Can you work these out from the model? Positions are in its coordinate system, mm. A direction names the side the tool comes from. Round coordinates to 2 decimals unless told otherwise and drop trailing zeros. Write each loop counter-clockwise with the first axis right and the second up, starting at its lowest first coordinate (ties: lowest second). Pieces come first, ordered by that corner, then holes. Notation, with made-up numbers: M 54,84.5 L 107,84.5 A28 ccw 107,123.5 Z; hole C 29,-15 d5. An arc over 180 degrees is marked long. Answer in a Markdown table with one row per item. Add a question column.
(1) For faces 4 (the face through (10, 0.675, 5)), 5 (the face through (0, -17, 12)), 6 (the face through (-9.4, 1.15, 10)), which set-ups out of +Z, -Z, +X, -X, +Y, -Y let a thin tool reach every point of the face, with its end or its side?
(2) If I drill on probe 1 along Z at (x, y) = (1.75, -4.5); probe 2 along Y at (x, z) = (6.5, 9.5); probe 3 along Y at (x, z) = (4.25, 12.75), over which ranges is the centre line in solid material (lowest first)?
(3) Suppose I cut it at A-A, the plane y = -1.75. Write out the boundary of the cut face in (x, z), then the cut area to 3 significant figures.
(4) I'm going to push flat-ended pins straight in: pin 1 (3.5 mm diameter, centred on x = 10.5, z = 2.5, fed in from -Y); pin 2 (1 mm diameter, centred on x = -6.5, z = 8, fed in from -Y); pin 3 (1.4 mm diameter, centred on x = -11, z = 2.5, fed in from -Y). Where does each tip first touch, or does it pass through?
(5) Suppose I cut it at C-C, the plane z = 1. Write out the boundary of the cut face in (x, y) (3 decimals).
(6) If we mould it in two halves opening along Z, with no side actions, what happens to faces 1 (the face through (0, 2.8, 2)), 2 (the face through (0, -9, 7)), 3 (the face through (0, -8, 14))? For each: released by +Z, released by -Z, zero draft, split by the parting line, or undercut.
(7) Suppose I cut it at D-D, the plane z = 6.25. Count the separate pieces of the cut face and the enclosed holes in it, then the cut area to 3 significant figures.
from build123d import *

# Parameters (mm, degrees)
F0_W     = 25.4
F0_H     = 5.6
F1_DEPTH = 10
F2_W     = 4.6
F2_H     = 1.35
F3_DEPTH = 10
F5_DEPTH = 5.6
F7_DEPTH = 25.4
F8_SIZE  = 0.4
F9_R     = 0.7
F10_R    = 0.29999


# Not quite as in the source:
# - a fillet or chamfer is up to 0.001 mm smaller than in the source, because OpenCascade refuses the exact size


with BuildPart() as f1:
    # F0 (on Top) → F1 (new body)
    with BuildSketch(Plane.XY):
        Rectangle(F0_W, F0_H)
    extrude(amount=F1_DEPTH)

    # F2 (on face) → F3 (cut, through all)
    with BuildSketch(Plane.XY.offset(10)):
        with Locations((-10.4, 0)):
            Rectangle(F2_W, F2_H)
        with Locations((10.4, 0)):
            Rectangle(F2_W, F2_H)
    extrude(amount=-F3_DEPTH, mode=Mode.SUBTRACT)

    # F4 (on face) → F5 (cut, through all)
    with BuildSketch(Plane.XZ.offset(2.8)):
        Polygon((6, 10), (-6, 10), (-1, 3), (1, 3), align=None)
    extrude(amount=-F5_DEPTH, mode=Mode.SUBTRACT)

    # F6 (on face) → F7 (join, through all)
    with BuildSketch(Plane(origin=(-12.7, 0, 0), x_dir=(0, -1, 0), z_dir=(-1, 0, 0))):
        Polygon((2.8, 2), (2.8, 0), (5.7319724348, 0), (15.8119724348, 12), (18.2, 12), (18.2, 14), (-1.8, 14), (-1.8, 12), (13.2, 12), (4.8, 2), align=None)
    extrude(amount=-F7_DEPTH)

    # F8
    f8_edges = [f1.edges().sort_by_distance(p)[0] for p in [
        (12.7, 0.675, 5),
        (12.7, -0.675, 5),
    ]]
    chamfer(f8_edges, length=F8_SIZE)

    # F9
    f9_edges = [f1.edges().sort_by_distance(p)[0] for p in [
        (0, -2.8, 2),
        (0, -4.8, 2),
        (0, -13.2, 12),
        (0, -15.811972, 12),
        (0, -5.731972, 0),
        (0, -18.2, 12),
        (0, -18.2, 14),
        (0, 1.8, 12),
        (0, 1.8, 14),
    ]]
    fillet(f9_edges, radius=F9_R)

    # F10 (radius 0.3 in the source; OpenCascade refuses exactly that, so slightly less here)
    f10_edges = [f1.edges().sort_by_distance(p)[0] for p in [
        (0, 2.8, 0),
        (9.35, 2.8, 10),
        (-9.35, 2.8, 10),
        (-10.4, 0.675, 0),
        (10.2, 0.675, 0),
        (10.2, -0.675, 0),
        (-10.4, -0.675, 0),
        (10.2, 0.675, 10),
        (10.2, -0.675, 10),
        (9.35, -2.8, 10),
        (-10.4, 0.675, 10),
        (-10.4, -0.675, 10),
        (-9.35, -2.8, 10),
        (3.5, 2.8, 6.5),
        (0, 2.8, 3),
        (-3.5, 2.8, 6.5),
        (0, -2.8, 3),
        (3.5, -2.8, 6.5),
        (-3.5, -2.8, 6.5),
    ]]
    fillet(f10_edges, radius=F10_R)


solid = f1.part
Calculated:
| question | item | result |
|---|---|---|
| 1 | face 4 | -Z, +X |
| 1 | face 5 | -Z, +X, -X, -Y |
| 1 | face 6 | +X, -X, +Y |
| 2 | probe 1 | 0 to 2, 12 to 14 |
| 2 | probe 2 | -13.71 to -11.1, -2.8 to 2.8 |
| 2 | probe 3 | -18.2 to 1.8 |
| 3 | outline | M -12.7,0 L 12.7,0 L 12.7,10 L 6,10 L 1,3 L -1,3 L -6,10 L -12.7,10 Z; M -12.7,12 L 12.7,12 L 12.7,14 L -12.7,14 Z |
| 3 | area | 256 mm² |
| 4 | pin 1 | y = -9.3 |
| 4 | pin 2 | y = -12.87 |
| 4 | pin 3 | y = -8.42 |
| 5 | outline | M -12.7,-6.572 L 12.7,-6.572 L 12.7,-1.075 L 12.3,-0.675 L 8.1,-0.675 L 8.1,0.675 L 12.3,0.675 L 12.7,1.075 L 12.7,2.8 L -12.7,2.8 L -12.7,0.675 L -8.1,0.675 L -8.1,-0.675 L -12.7,-0.675 Z |
| 6 | face 1 | zero draft |
| 6 | face 2 | undercut |
| 6 | face 3 | released by +Z |
| 7 | separate pieces | 3 |
| 7 | enclosed holes | 0 |
| 7 | area | 159 mm² |
